Work out the finished part from the listing and answer in its coordinate system (mm). Coordinates: 2 decimals unless noted, no trailing zeros. Write each loop counter-clockwise with the first axis right and the second up, starting at its lowest first coordinate (ties: lowest second). Pieces come first, ordered by that corner, then holes. Notation, with made-up numbers: (-35.5, 86.5) - (11.5, 86.5) arc R20 ccw to (11.5, 116.5) - close; hole circle Ø4 at (84, 5.5). An arc over 180 degrees is marked (long way). Answer as a JSON object with one key per item and string values. Group by question number.
from build123d import *

# Parameters (mm, degrees)
SKETCH1_R             = 35.015
SKETCH1_R_2           = 2.555
BOSS_EXTRUDE1_DEPTH   = 2
CHAMFER1_SIZE         = 0.5
M4X0_7_TAPPED_HOLE1_D = 3.3


with BuildPart() as part:
    # Sketch1 → Boss-Extrude1 (new body)
    with BuildSketch(Plane(origin=(0, 0, 0), x_dir=(1, 0, 0), z_dir=(0, 1, 0))):
        Circle(SKETCH1_R)
        Circle(SKETCH1_R_2, mode=Mode.SUBTRACT)
    extrude(amount=BOSS_EXTRUDE1_DEPTH)

    # Chamfer1
    chamfer1_edges = [part.edges().sort_by_distance(p)[0] for p in [
        (-35.015, 2, 0),
    ]]
    chamfer(chamfer1_edges, length=CHAMFER1_SIZE)

    # M4x0.7 Tapped Hole1 (through all)
    with Locations(Plane(origin=(3.342611255, 2, 28.08606327), x_dir=(0, 0, 1), z_dir=(0, 1, 0))):
        with Locations((0, 0), (-24.743452015, -31.428674525), (-50.82191635, 8.193461939), (-31.428674525, 24.743452015)):
            Hole(M4X0_7_TAPPED_HOLE1_D / 2)


solid = part.part
Q1. Section A-A on z = 0 is taken. Determine the outline of the cut face in (x, y) (3 decimals), plus the area to 3 significant figures.
Q2. For a pull along X with two mould halves and no side action, classify faces 1 (the face through (0, 2, 7)), 2 (the face through (33.398, 0.74, -10.518)), 3 (the face through (29.722, 0.986, -3.128)) as +X half, -X half, draft (parallel to the pull), parting line (faces both ways), or undercut.
Q3. Consider L1, parallel to Z at x = 0, y = 0.7 (3 decimals); L2, parallel to X at y = 1.75, z = 3; L3, parallel to Z at x = 18.5, y = 1.05. Determine where each line is inside the solid, lowest interval first. Write a range as from..to.
Q4. Section C-C on y = 1.05 is taken. Determine the outline of the cut face in (x, z) (3 decimals).
Q5. Section B-B on x = 0 is taken. Determine the outline of the cut face in (y, z) (3 decimals), plus the area to 3 significant figures.
Q6. Flat-ended cylindrical pins translate along their axes: pin 1 Ø3 at (x, z) = (3.34, 28.09) entering from +Y; pin 2 Ø1 at (x, y) = (17.5, 0.5) entering from +Z; pin 3 Ø1 at (y, z) = (1.5, 2.5) entering from +X. Find the tip coordinate at first contact, or state that the pin passes through.
Numbers:
{
 "1": {"outline": "(-35.015, 0) - (-2.555, 0) - (-2.555, 2) - (-34.515, 2) - (-35.015, 1.5) - close; (2.555, 0) - (35.015, 0) - (35.015, 1.5) - (34.515, 2) - (2.555, 2) - close", "area": "130 mm²"},
 "2": {"face 1": "draft", "face 2": "parting line", "face 3": "undercut"},
 "3": {"L1": "z = -35.015..-2.555, 2.555..35.015", "L2": "x = -34.64..-29.7, -26.47..34.64", "L3": "z = -29.73..29.73"},
 "4": {"outline": "circle Ø70.03 at (0, 0); hole circle Ø3.3 at (-28.086, 3.343); hole circle Ø5.11 at (0, 0); hole circle Ø3.3 at (3.343, 28.086); hole circle Ø3.3 at (11.536, -22.736); hole circle Ø3.3 at (28.086, -3.343)"},
 "5": {"outline": "(0, -35.015) - (1.5, -35.015) - (2, -34.515) - (2, -2.555) - (0, -2.555) - close; (0, 2.555) - (2, 2.555) - (2, 34.515) - (1.5, 35.015) - (0, 35.015) - close", "area": "130 mm²"},
 "6": {"pin 1": "passes through", "pin 2": "stops at z = 30.61", "pin 3": "stops at x = 34.96"}
}
